from build123d import *

# Parameters (mm, degrees)
SKETCH1_W           = 230
SKETCH1_H           = 95
BOSS_EXTRUDE1_DEPTH = 3
SKETCH2_W           = 205
SKETCH2_H           = 80
CUT_EXTRUDE1_DEPTH  = 1.5
SKETCH3_W           = 230
SKETCH3_H           = 95
SKETCH3_W_2         = 224
SKETCH3_H_2         = 89
BOSS_EXTRUDE2_DEPTH = 70
SKETCH4_R           = 4.5
CUT_EXTRUDE2_DEPTH  = 3
SKETCH5_R           = 4.5
CUT_EXTRUDE3_DEPTH  = 3


with BuildPart() as part:
    # Sketch1 → Boss-Extrude1 (new body)
    with BuildSketch(Plane(origin=(0, 0, 0), x_dir=(1, 0, 0), z_dir=(0, 1, 0))):
        Rectangle(SKETCH1_W, SKETCH1_H)
    extrude(amount=BOSS_EXTRUDE1_DEPTH)

    # Sketch2 → Cut-Extrude1 (cut)
    with BuildSketch(Plane(origin=(0, 3, 0), x_dir=(1, 0, 0), z_dir=(0, 1, 0))):
        Rectangle(SKETCH2_W, SKETCH2_H)
    extrude(amount=-CUT_EXTRUDE1_DEPTH, mode=Mode.SUBTRACT)

    # Sketch3 → Boss-Extrude2 (add)
    with BuildSketch(Plane(origin=(0, 3, 0), x_dir=(1, 0, 0), z_dir=(0, 1, 0))):
        Rectangle(SKETCH3_W, SKETCH3_H)
        Rectangle(SKETCH3_W_2, SKETCH3_H_2, mode=Mode.SUBTRACT)
    extrude(amount=BOSS_EXTRUDE2_DEPTH)

    # Sketch4 → Cut-Extrude2 (cut)
    with BuildSketch(Plane.XY.offset(47.5)):
        with Locations((95, 28)):
            Circle(SKETCH4_R)
        with Locations((71.25, 28)):
            Circle(SKETCH4_R)
        with Locations((47.5, 28)):
            Circle(SKETCH4_R)
        with Locations((23.75, 28)):
            Circle(SKETCH4_R)
        with Locations((0, 28)):
            Circle(SKETCH4_R)
        with Locations((-23.75, 28)):
            Circle(SKETCH4_R)
        with Locations((-47.5, 28)):
            Circle(SKETCH4_R)
        with Locations((-71.25, 28)):
            Circle(SKETCH4_R)
        with Locations((-95, 28)):
            Circle(SKETCH4_R)
        with BuildLine():
            Line((-101.5, 62.5), (-101.5, 43.5))
            Line((-101.5, 43.5), (-88.5, 43.5))
            Line((-88.5, 43.5), (-88.5, 62.5))
            ThreePointArc((-88.5, 62.5), (-95, 69), (-101.5, 62.5))
        make_face()
        with BuildLine():
            Line((-77.75, 62.5), (-77.75, 43.5))
            Line((-77.75, 43.5), (-64.75, 43.5))
            Line((-64.75, 43.5), (-64.75, 62.5))
            ThreePointArc((-64.75, 62.5), (-71.25, 69), (-77.75, 62.5))
        make_face()
        with BuildLine():
            Line((-54, 62.5), (-54, 43.5))
            Line((-54, 43.5), (-41, 43.5))
            Line((-41, 43.5), (-41, 62.5))
            ThreePointArc((-41, 62.5), (-47.5, 69), (-54, 62.5))
        make_face()
        with BuildLine():
            Line((-30.25, 62.5), (-30.25, 43.5))
            Line((-30.25, 43.5), (-17.25, 43.5))
            Line((-17.25, 43.5), (-17.25, 62.5))
            ThreePointArc((-17.25, 62.5), (-23.75, 69), (-30.25, 62.5))
        make_face()
        with BuildLine():
            Line((-6.5, 62.5), (-6.5, 43.5))
            Line((-6.5, 43.5), (6.5, 43.5))
            Line((6.5, 43.5), (6.5, 62.5))
            ThreePointArc((6.5, 62.5), (0, 69), (-6.5, 62.5))
        make_face()
        with BuildLine():
            Line((17.25, 62.5), (17.25, 43.5))
            Line((17.25, 43.5), (30.25, 43.5))
            Line((30.25, 43.5), (30.25, 62.5))
            ThreePointArc((30.25, 62.5), (23.75, 69), (17.25, 62.5))
        make_face()
        with BuildLine():
            Line((41, 62.5), (41, 43.5))
            Line((41, 43.5), (54, 43.5))
            Line((54, 43.5), (54, 62.5))
            ThreePointArc((54, 62.5), (47.5, 69), (41, 62.5))
        make_face()
        with BuildLine():
            Line((64.75, 62.5), (64.75, 43.5))
            Line((64.75, 43.5), (77.75, 43.5))
            Line((77.75, 43.5), (77.75, 62.5))
            ThreePointArc((77.75, 62.5), (71.25, 69), (64.75, 62.5))
        make_face()
    extrude(amount=-CUT_EXTRUDE2_DEPTH, mode=Mode.SUBTRACT)

    # Sketch5 → Cut-Extrude3 (cut)
    with BuildSketch(Plane(origin=(0, 0, -47.5), x_dir=(-1, 0, 0), z_dir=(0, 0, -1))):
        with Locations((-100, 23)):
            Circle(SKETCH5_R)
        with Locations((-70, 23)):
            Circle(SKETCH5_R)
        with Locations((-40, 23)):
            Circle(SKETCH5_R)
    extrude(amount=-CUT_EXTRUDE3_DEPTH, mode=Mode.SUBTRACT)


solid = part.part
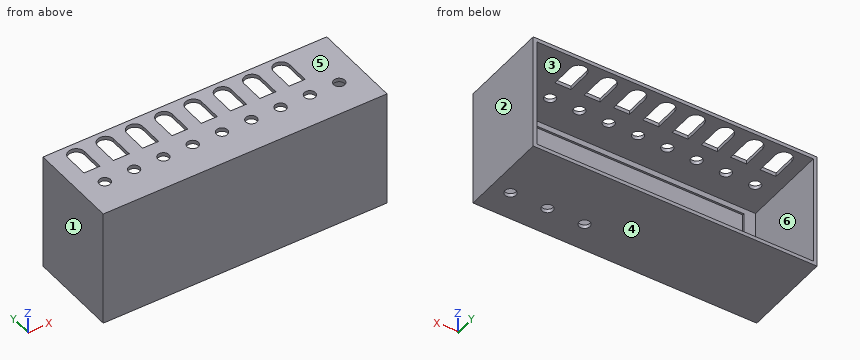
Can you work these out from the model? Positions are in its coordinate system, mm. Face numbers are marked on the shaded views. A direction names the side the tool comes from. Give positions to 0.01 mm unless a question says otherwise; leave off trailing zeros. Order: outer loops, then holes, each group sorted by start corner. A loop starts at its lowest first (then second) coordinate and runs counter-clockwise, first axis right, second up. Notation, with made-up numbers: M 48.25,73.25 L 60.25,73.25 A31 ccw 60.25,110.25 Z; hole C 18,-30 d11. An arc over 180 degrees is marked long. One line per question, with ' | ' between items.
Item 1: For the marked faces 5 and 6, which set-ups out of +Z, -Z, +X, -X, +Y, -Y let a thin tool reach every point of the face, with its end or its side?
Answer block:
face 5: +Z, +X, -X, +Y, -Y | face 6: +Y
Item 2: Suppose I cut it at C-C, the plane y = 65.5. Give the number of separate pieces and of enclosed holes in the cut face, then the cut area to 3 significant figures.
Answer block:
separate pieces: 8 | enclosed holes: 0 | area: 1,640 mm2
Item 3: Suppose I cut it at A-A, the plane x = -95. Write out the boundary of the cut face in (y, z), then the cut area to 4 significant figures.
Answer block:
outline: M 0,-47.5 L 73,-47.5 L 73,-44.5 L 3,-44.5 L 3,-40 L 1.5,-40 L 1.5,40 L 3,40 L 3,44.5 L 23.5,44.5 L 23.5,47.5 L 0,47.5 Z; M 32.5,44.5 L 43.5,44.5 L 43.5,47.5 L 32.5,47.5 Z; M 69,44.5 L 73,44.5 L 73,47.5 L 69,47.5 Z | area: 481.5 mm2
Item 4: Suppose I cut it at B-B, the plane z = -28. Write out the boundary of the cut face in (x, y).
Answer block:
outline: M -115,0 L 115,0 L 115,73 L 112,73 L 112,3 L 102.5,3 L 102.5,1.5 L -102.5,1.5 L -102.5,3 L -112,3 L -112,73 L -115,73 Z
Item 5: I'm going to push flat-ended pins straight in: pin 1 Ø3 at (x, y) = (19, 56) entering from +Z; pin 2 Ø8 at (x, z) = (38, -22) entering from -Y; pin 3 Ø5 at (x, z) = (72, 1.5) entering from +Y. Where does each tip first touch, or does it pass through?
Answer block:
pin 1: stops at z = -44.5 | pin 2: stops at y = 0 | pin 3: stops at y = 1.5
Item 6: Please list where these lines run through material, in increasing order: L1, parallel to Y at x = -71, z = 45; L2, parallel to X at y = 51.5, z = 43; L3, parallel to Y at x = 40, z = -45.7.
Answer block:
L1: y = 0 to 23.51, 32.49 to 43.5, 69 to 73 | L2: x = -115 to -112, 112 to 115 | L3: y = 0 to 18.5, 27.5 to 73
Item 7: We'd pull the mould along X, two halves only. Please class the marked faces 1, 2, 3 and 4: released by +X, released by -X, zero draft, split by the parting line, or undercut.
Answer block:
face 1: released by -X | face 2: released by +X | face 3: undercut | face 4: zero draft
